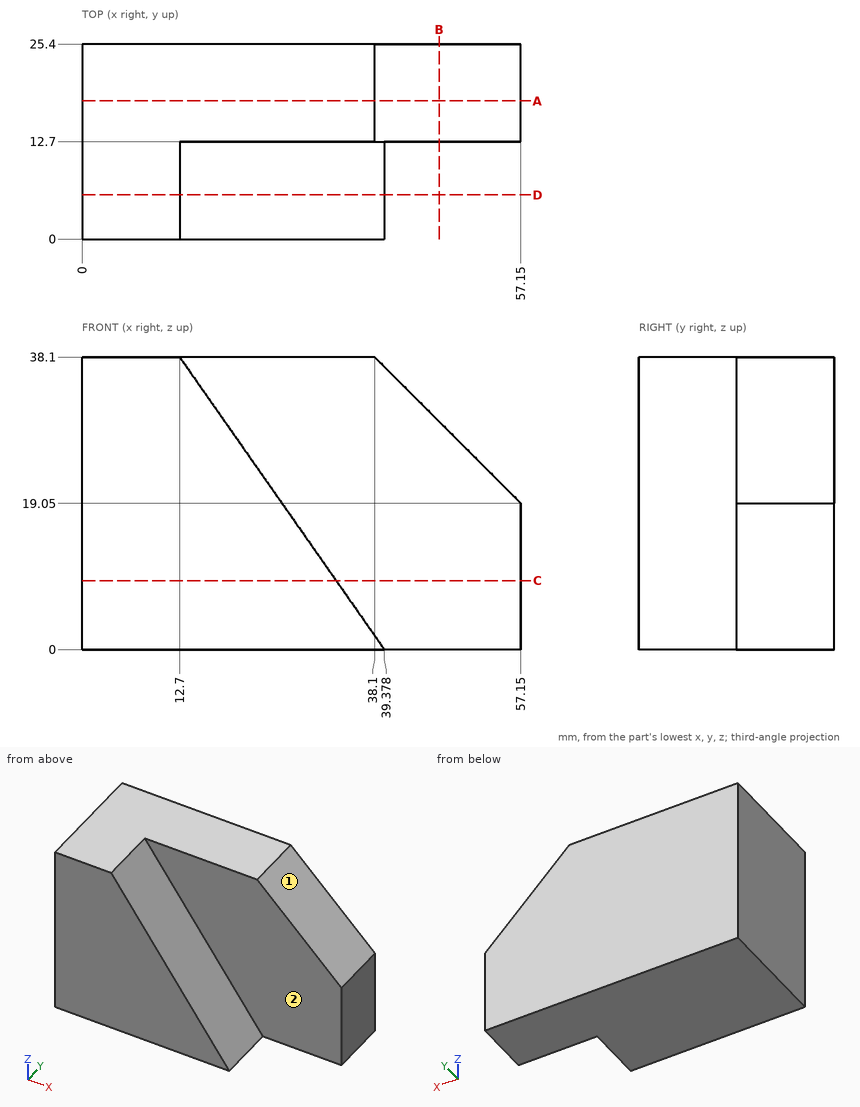
Drawing for the job (mm, zero at the part's lowest x, y, z). A direction names the side the tool comes from. Coordinates: 2 decimals unless noted, no trailing zeros. Order: outer loops, then holes, each group sorted by start corner. A loop starts at its lowest first (then second) coordinate and runs counter-clockwise, first axis right, second up.
Item 1: 3-axis set-ups, long thin cutter, end or side, ignore diameter. For the marked faces 1 and 2: which of +Z, -Z, +X, -X, +Y, -Y reach the whole face in a straight line?
Check sheet entries:
face 1: +Z, +X, +Y, -Y
face 2: +Z, +X, -Y
Item 2: Band-saw the part on C-C on z = 9. List the corners of the cut face in (x, y).
Check sheet entries:
outline: (0, 0) - (33.08, 0) - (33.08, 12.7) - (57.15, 12.7) - (57.15, 25.4) - (0, 25.4) - close
Item 3: Drill centre lines: L1, parallel to Y at x = 28, z = 27; L2, parallel to Z at x = 24, y = 7.25; L3, parallel to X at y = 6.25, z = 23. Where is each one in solid material? Low to high.
Check sheet entries:
L1: y = 12.7 to 25.4
L2: z = 0 to 21.96
L3: x = 0 to 23.27
Item 4: Pin check, flat tips, straight feed: pin 1 Ø4 at (y, z) = (3.5, 18.5) entering from +X; pin 2 Ø5 at (y, z) = (8, 29.5) entering from +X; pin 3 Ø4 at (x, y) = (45.5, 12) entering from +Z. Stop position of each tip, or through.
Check sheet entries:
pin 1: stops at x = 27.82
pin 2: stops at x = 20.47
pin 3: stops at z = 32.57
Item 5: Band-saw the part on A-A on y = 18. List the corners of the cut face in (x, z).
Check sheet entries:
outline: (0, 0) - (57.15, 0) - (57.15, 19.05) - (38.1, 38.1) - (0, 38.1) - close
Item 6: Band-saw the part on D-D on y = 5.75. List the corners of the cut face in (x, z).
Check sheet entries:
outline: (0, 0) - (39.38, 0) - (12.7, 38.1) - (0, 38.1) - close
Item 7: Band-saw the part on B-B on x = 46.5. List the corners of the cut face in (y, z).
Check sheet entries:
outline: (12.7, 0) - (25.4, 0) - (25.4, 29.7) - (12.7, 29.7) - close
